from build123d import *

# Parameters (mm, degrees)
SKETCH1_R           = 508
SKETCH1_R_2         = 63.5
BOSS_EXTRUDE1_DEPTH = 38.1
FILLET1_R           = 6.35


with BuildPart() as part:
    # Sketch1 → Boss-Extrude1 (new, symmetric)
    with BuildSketch(Plane.XY):
        with Locations(Location((0, 0, 0), (0, 0, 180))):
            Circle(SKETCH1_R)
        with Locations(Location((0, 0, 0), (0, 0, 180))):
            Circle(SKETCH1_R_2, mode=Mode.SUBTRACT)
        with Locations(Location((0, 355.6, 0), (0, 0, 180))):
            Circle(SKETCH1_R_2, mode=Mode.SUBTRACT)
    extrude(amount=BOSS_EXTRUDE1_DEPTH, both=True)

    # Fillet1
    fillet1_edges = [part.edges().sort_by_distance(p)[0] for p in [
        (508, 0, -38.1),
        (508, 0, 38.1),
    ]]
    fillet(fillet1_edges, radius=FILLET1_R)


solid = part.part
Geometry check sheet. Reference: the model listing, model coordinates, mm. Give positions to 0.01 mm unless a question says otherwise; leave off trailing zeros. Write each loop counter-clockwise with the first axis right and the second up, starting at its lowest first coordinate (ties: lowest second). Pieces come first, ordered by that corner, then holes.
1) Cross-section at A-A (y = 0). Record the boundary of the cut face in (x, z), plus the area to 3 significant figures.
Values follow:
outline: (-508, -31.75) arc R6.35 ccw to (-501.65, -38.1) - (-63.5, -38.1) - (-63.5, 38.1) - (-501.65, 38.1) arc R6.35 ccw to (-508, 31.75) - close; (63.5, -38.1) - (501.65, -38.1) arc R6.35 ccw to (508, -31.75) - (508, 31.75) arc R6.35 ccw to (501.65, 38.1) - (63.5, 38.1) - close
area: 67,700 mm2
2) Thickness scan on line 1 (Y direction, x = 0, z = 5); line 2 (X direction, y = 355.6, z = -13); line 3 (X direction, y = 344, z = 15). Record the ranges inside material, lowest first.
Values follow:
line 1: y = -508 to -63.5, 63.5 to 292.1, 419.1 to 508
line 2: x = -362.78 to -63.5, 63.5 to 362.78
line 3: x = -373.8 to -62.43, 62.43 to 373.8
3) Cross-section at B-B (x = 0). Record the boundary of the cut face in (y, z).
Values follow:
outline: (-508, -31.75) arc R6.35 ccw to (-501.65, -38.1) - (-63.5, -38.1) - (-63.5, 38.1) - (-501.65, 38.1) arc R6.35 ccw to (-508, 31.75) - close; (63.5, -38.1) - (292.1, -38.1) - (292.1, 38.1) - (63.5, 38.1) - close; (419.1, -38.1) - (501.65, -38.1) arc R6.35 ccw to (508, -31.75) - (508, 31.75) arc R6.35 ccw to (501.65, 38.1) - (419.1, 38.1) - close
4) Go/stop test with flat-tipped pins: pin 1 Ø6 at (x, z) = (-243.5, -23.5) entering from -Y; pin 2 Ø5 at (x, z) = (294.5, 10.5) entering from +Y; pin 3 Ø1.5 at (x, z) = (53, 25.5) entering from +Y. Record where each tip stops, or that it passes through.
Values follow:
pin 1: stops at y = -447.46
pin 2: stops at y = 415.69
pin 3: stops at y = 505.31
5) Release check for a two-part mould opening along Y. For faces 1 (the face through (-104, -7, 38.1)), 2 (the face through (110.12, 495.92, 0.44)), 3 (the face through (13.77, 61.99, -0.53)) record: released by +Y, released by -Y, zero draft, split by the parting line, or undercut.
Values follow:
face 1: zero draft
face 2: split by the parting line
face 3: undercut
6) Cross-section at C-C (z = 18). Record the boundary of the cut face in (x, y).
Values follow:
outline: circle Ø1016 at (0, 0); hole circle Ø127 at (0, 0); hole circle Ø127 at (0, 355.6)
